```python
from build123d import *

# Parameters (mm, degrees)
SKETCH1_W               = 92.0242
SKETCH1_H               = 20.32
BOSS_EXTRUDE1_DEPTH     = 444.5
SKETCH2_W               = 54.356
SKETCH2_H               = 15.3416
SKETCH2_W_2             = 16.3449
SKETCH2_H_2             = 17.8308
CUT_EXTRUDE1_DEPTH      = 445.5
SKETCH3_W               = 33.274
SKETCH3_H               = 76.2
CUT_EXTRUDE2_DEPTH      = 21.32
SKETCH4_W               = 3.5052
SKETCH4_H               = 63.5
CUT_EXTRUDE3_DEPTH      = 12.7
CUT_EXTRUDE5_DEPTH      = 76.6793001
SKETCH6_R               = 3.175
CUT_EXTRUDE6_DEPTH      = 76.6793001
SKETCH7_R               = 1.764906423
CUT_EXTRUDE7_DEPTH      = 76.6793001
SKETCH9_R               = 3.175
CUT_EXTRUDE8_DEPTH      = 47.0121001
CUT_EXTRUDE8_DEPTH_BACK = 47.0121001


with BuildPart() as part:
    # Sketch1 → Boss-Extrude1 (new body)
    with BuildSketch(Plane.XY):
        with Locations((0, -10.16)):
            Rectangle(SKETCH1_W, SKETCH1_H)
    extrude(amount=-BOSS_EXTRUDE1_DEPTH)

    # Sketch2 → Cut-Extrude1 (cut, through all)
    with BuildSketch(Plane.XY):
        with Locations((0, -10.16)):
            Rectangle(SKETCH2_W, SKETCH2_H)
        with Locations((37.83965, -11.4046)):
            Rectangle(SKETCH2_W_2, SKETCH2_H_2)
        with Locations((-37.83965, -11.4046)):
            Rectangle(SKETCH2_W_2, SKETCH2_H_2)
    extrude(amount=-CUT_EXTRUDE1_DEPTH, mode=Mode.SUBTRACT)

    # Sketch3 → Cut-Extrude2 (cut, through all)
    with BuildSketch(Plane(origin=(0, 0, 0), x_dir=(1, 0, 0), z_dir=(0, 1, 0))):
        with BuildLine():
            Line((-46.0121, 0), (-28.575, 0))
            add(Edge.make_bspline(
                [(-28.575, 0), (-35.717859011, 0), (-38.245794082, 5.707856621), (-38.842625262, 8.197153509)],
                knots=[0, 0, 0, 0, 1, 1, 1, 1], degree=3))
            Line((-38.842625262, 8.197153509), (-46.0121, 38.1))
            Line((-46.0121, 38.1), (-46.0121, 0))
        make_face()
        with BuildLine():
            add(Edge.make_bspline(
                [(28.575, 0), (35.717859011, 0), (38.245794082, 5.707856621), (38.842625262, 8.197153509)],
                knots=[0, 0, 0, 0, 1, 1, 1, 1], degree=3))
            Line((28.575, 0), (46.0121, 0))
            Line((46.0121, 0), (46.0121, 38.1))
            Line((46.0121, 38.1), (38.842625262, 8.197153509))
        make_face()
        with BuildLine():
            Line((46.0121, 444.5), (28.6258, 444.5))
            add(Edge.make_bspline(
                [(28.6258, 444.5), (32.693382337, 426.337896511), (31.854875968, 406.755772808), (43.153705429, 392.326383256)],
                knots=[0, 0, 0, 0, 0.951264786, 0.951264786, 0.951264786, 0.951264786], degree=3))
            ThreePointArc((43.153705429, 392.326383256), (44.408270339, 390.171508327), (45.032534863, 387.757442695))
            Line((45.032534863, 387.757442695), (46.0121, 379.348138392))
            Line((46.0121, 379.348138392), (46.0121, 444.5))
        make_face()
        with Locations((0, 406.4)):
            Rectangle(SKETCH3_W, SKETCH3_H)
        with BuildLine():
            add(Edge.make_bspline(
                [(-28.6258, 444.5), (-32.693382337, 426.337896511), (-31.854875968, 406.755772808), (-43.153705429, 392.326383256)],
                knots=[0, 0, 0, 0, 0.951264786, 0.951264786, 0.951264786, 0.951264786], degree=3))
            Line((-28.6258, 444.5), (-46.0121, 444.5))
            Line((-46.0121, 444.5), (-46.0121, 379.348138392))
            Line((-46.0121, 379.348138392), (-45.032534863, 387.757442695))
            ThreePointArc((-45.032534863, 387.757442695), (-44.408270339, 390.171508327), (-43.153705429, 392.326383256))
        make_face()
    extrude(amount=-CUT_EXTRUDE2_DEPTH, mode=Mode.SUBTRACT)

    # Sketch4 → Cut-Extrude3 (cut)
    with BuildSketch(Plane(origin=(0, 0, 0), x_dir=(1, 0, 0), z_dir=(0, 1, 0))):
        with Locations((20.4724, 31.75)):
            Rectangle(SKETCH4_W, SKETCH4_H)
        with Locations((-20.4724, 31.75)):
            Rectangle(SKETCH4_W, SKETCH4_H)
    extrude(amount=-CUT_EXTRUDE3_DEPTH, mode=Mode.SUBTRACT)

    # Sketch5 → Cut-Extrude5 (cut, through all)
    with BuildSketch(Plane(origin=(29.6672, 0, 0), x_dir=(0, 0, -1), z_dir=(1, 0, 0))):
        Polygon((0.046334806, -2.4892), (-3.084672114, 2.933863065), (-3.084672114, -20.32), (0.046334806, -20.32), align=None)
        Polygon((10.340951986, -20.32), (0.046334806, -2.4892), (0.046334806, -20.32), align=None)
    extrude(amount=-CUT_EXTRUDE5_DEPTH, mode=Mode.SUBTRACT)

    # Sketch6 → Cut-Extrude6 (cut, through all)
    with BuildSketch(Plane(origin=(29.6672, 0, 0), x_dir=(0, 0, -1), z_dir=(1, 0, 0))):
        with Locations((23.09476437, -11.4046)):
            Circle(SKETCH6_R)
        with Locations((51.66976437, -11.4046)):
            Circle(SKETCH6_R)
    extrude(amount=-CUT_EXTRUDE6_DEPTH, mode=Mode.SUBTRACT)

    # Sketch7 → Cut-Extrude7 (cut, through all)
    with BuildSketch(Plane(origin=(29.6672, 0, 0), x_dir=(0, 0, -1), z_dir=(1, 0, 0))):
        with Locations((368.3, -6.418973604)):
            Circle(SKETCH7_R)
    extrude(amount=-CUT_EXTRUDE7_DEPTH, mode=Mode.SUBTRACT)

    # Sketch9 → Cut-Extrude8 (cut, two sides)
    with BuildSketch(Plane(origin=(0, 0, 0), x_dir=(0, 0, -1), z_dir=(1, 0, 0))) as cut_extrude8_sk:
        with Locations((427.0375, -10.16)):
            Circle(SKETCH9_R)
    extrude(amount=CUT_EXTRUDE8_DEPTH, mode=Mode.SUBTRACT)
    extrude(cut_extrude8_sk.sketch, amount=-CUT_EXTRUDE8_DEPTH_BACK, mode=Mode.SUBTRACT)


solid = part.part
```
Here's how the part is built. I have some questions about the finished solid (model axes, mm). A direction names the side the tool comes from. Coordinates: 2 decimals unless noted, no trailing zeros. Order: outer loops, then holes, each group sorted by start corner. A loop starts at its lowest first (then second) coordinate and runs counter-clockwise, first axis right, second up. Notation, with made-up numbers: M 74.5,40.25 L 102.5,40.25 A23 ccw 102.5,71.25 Z; hole C -13.5,22.25 d6. An arc over 180 degrees is marked long. Answer as a JSON object with one key per item and string values. Group by question number.
(1) Suppose I cut it at A-A, the plane z = -349. Please give me the cut outline in (x, y), then the cut area to 3 significant figures.
(2) I need wall thicknesses on probe 1 along Y at (x, z) = (27, -368); probe 2 along X at (y, z) = (-10.75, -71); probe 3 along Z at (x, y) = (-28, -11.75). Which ranges of each line are inside material? Lowest first, please.
(3) Suppose I cut it at B-B, the plane x = 5. Please give me the cut outline in (y, z), then the cut area to 3 significant figures.
(4) If we mould it in two halves opening along X, with no side actions, what happens to faces 4 (the face through (29.667, -12, -217)), 5 (the face through (38, -2.489, -217)), 6 (the face through (-27.178, -10, -219))? For each: released by +X, released by -X, zero draft, split by the parting line, or undercut.
(5) For pin 1 (2.5 mm diameter, centred on x = 20, y = -1, fed in from +Z); pin 2 (8.5 mm diameter, centred on y = -11.4, z = -23.09, fed in from +X); pin 3 (2.5 mm diameter, centred on y = -1, z = -417.5, fed in from -X), each with a flat end and sliding along its axis, tell me the tip position at first contact or that it passes through.
(6) Which directions (+Z, -Z, +X, -X, +Y, -Y) give clear straight access to the entire face, cutting with the end or side of a thin tool? Please do faces 1 (the face through (0, -17.831, -224)), 2 (the face through (-38, -2.489, -217)), 3 (the face through (0, -20.32, -224)).
Values found:
{
 "1": {"outline": "M -46.01,-2.49 L -29.67,-2.49 L -29.67,-20.32 L 29.67,-20.32 L 29.67,-2.49 L 46.01,-2.49 L 46.01,0 L -46.01,0 Z; hole M -27.18,-17.83 L 27.18,-17.83 L 27.18,-2.49 L -27.18,-2.49 Z", "area": "453 mm^2"},
 "2": {"probe 1": "y = -20.32 to -17.83, -2.49 to 0", "probe 2": "x = -29.67 to -27.18, 27.18 to 29.67", "probe 3": "z = -444.5 to -429.79, -424.29 to -54.83, -48.51 to -26.25, -19.94 to -5.39"},
 "3": {"outline": "M -20.32,-368.3 L -17.83,-368.3 L -17.83,-8.9 L -20.32,-10.34 Z; M -2.49,-368.3 L 0,-368.3 L 0,0 L -2.41,0 L -2.49,-0.05 Z", "area": "1,810 mm^2"},
 "4": {"face 4": "released by +X", "face 5": "zero draft", "face 6": "undercut"},
 "5": {"pin 1": "stops at z = -63.5", "pin 2": "stops at x = 29.67", "pin 3": "stops at x = -33.33"},
 "6": {"face 1": "+Z, -Z", "face 2": "+Z, -Z, -X, -Y", "face 3": "+Z, -Z, +X, -X, -Y"}
}
